Part model, mm, in its own coordinate system. A direction names the side the tool comes from. Round coordinates to 2 decimals unless told otherwise and drop trailing zeros. Loops run counter-clockwise (first coordinate to the right, second up) from the corner with the lowest first, then second, coordinate; pieces in that order, holes last.
(1) Cut at B-B on z = 94. List the corners of the cut face in (x, y).
(2) Flat gauge pins, fed straight in: pin 1 (2 mm diameter, centred on y = 14, z = 63.5, fed in from +X); pin 2 (5.5 mm diameter, centred on x = 0, y = 22.5, fed in from -Z); pin 3 (1 mm diameter, centred on x = -10.5, z = 75.5, fed in from +Y); pin 4 (2 mm diameter, centred on x = -1, z = 33.5, fed in from -Y). Where does each tip first touch, or does it go through?
(3) Mould opens along X. For faces 5 (the face through (-16.52, -11.57, 103.02)), 6 (the face through (-20, -11, 65)), 7 (the face through (-0.867, -3.905, 69.02)), 8 (the face through (18.28, -8.52, 103.02)) say: +X half, -X half, draft (parallel to the pull), parting line (faces both ways), or undercut.
(4) Tool access for faces 1 (the face through (-1.76, 20.1, 103.02)), 2 (the face through (0, 24, 65)), 3 (the face through (16.1, -11.3, 103)), 4 (the face through (1.74, 19.65, 103.02)): list every direction of +Z, -Z, +X, -X, +Y, -Y with a clear straight run to the whole face (end or side of a thin tool).
(5) Cut at C-C on x = 11.5. List the corners of the cut face in (y, z).
(6) Cut at D-D on y = 5.5. List the corners of the cut face in (x, z), then the cut area to 3 significant figures.
(7) Cut at A-A on y = -11.5. List the corners of the cut face in (x, z).
(8) Probe probe 1 along X at (y, z) = (-14, 124); probe 2 along Z at (x, y) = (-1.5, 30); probe 3 along X at (y, z) = (-9, 80). List the from-to ranges inside material, lowest first.
from build123d import *

# Parameters (mm, degrees)
SKETCH1_R           = 4
BOSS_EXTRUDE1_DEPTH = 140
BOSS_EXTRUDE2_DEPTH = 75


with BuildPart() as part:
    # Sketch1 → Boss-Extrude1 (new body)
    with BuildSketch(Plane.XY):
        Circle(SKETCH1_R)
    extrude(amount=BOSS_EXTRUDE1_DEPTH)

    # Sketch2 → Boss-Extrude2 (add)
    with BuildSketch(Plane.XY.offset(140)):
        Polygon((2.5, 35.872983346), (-2.5, 35.872983346), (-1, 3.872983346), (1, 3.872983346), align=None)
        Polygon((32.316914887, -15.771428164), (3.854101966, -1.070466269), (2.854101966, -2.802517077), (29.816914887, -20.101555183), align=None)
        Polygon((-29.816914887, -20.101555183), (-2.854101966, -2.802517077), (-3.854101966, -1.070466269), (-32.316914887, -15.771428164), align=None)
    extrude(amount=-BOSS_EXTRUDE2_DEPTH)


solid = part.part
Final values:
1. outline: (-32.32, -15.77) - (-29.82, -20.1) - (-2.85, -2.8) arc R4 ccw to (2.85, -2.8) - (29.82, -20.1) - (32.32, -15.77) - (3.85, -1.07) arc R4 ccw to (1, 3.87) - (2.5, 35.87) - (-2.5, 35.87) - (-1, 3.87) arc R4 ccw to (-3.85, -1.07) - close
2. pin 1: passes through
2. pin 2: stops at z = 65
2. pin 3: stops at y = -4.24
2. pin 4: stops at y = -4
3. face 5: undercut
3. face 6: draft
3. face 7: undercut
3. face 8: +X half
4. face 1: +Z, -Z, -X
4. face 2: -Z, +X, -X, +Y
4. face 3: +Z, -Z, -Y
4. face 4: +Z, -Z, +X
5. outline: (-8.35, 65) - (-5.02, 65) - (-5.02, 140) - (-8.35, 140) - close
6. outline: (-1.08, 65) - (1.08, 65) - (1.08, 140) - (-1.08, 140) - close
6. area: 161 mm2
7. outline: (-24.05, 65) - (-16.41, 65) - (-16.41, 140) - (-24.05, 140) - close; (16.41, 65) - (24.05, 65) - (24.05, 140) - (16.41, 140) - close
8. probe 1: x = -28.89 to -20.31, 20.31 to 28.89
8. probe 2: z = 65 to 140
8. probe 3: x = -19.21 to -12.51, 12.51 to 19.21
